Geometry: see drawing. Coordinates: mm, zero at the bounding-box minimum. A direction names the side the tool comes from. Coordinates: 2 decimals unless noted, no trailing zeros. Loops run counter-clockwise (first coordinate to the right, second up) from the corner with the lowest first, then second, coordinate; pieces in that order, holes last. Notation, with made-up numbers: (-9, -34.5) -> (46, -34.5) arc R14 ccw to (46, -20.5) -> close; hole circle Ø4 at (-13.75, 59). An arc over 180 degrees is marked (long way). One line per item, written item: value. Start each with the question number.
Item 1: Section query A-A on z = 3.35. Return loops of the section in (x, y).
Item 2: Ray query, probe 1 along Y at (x, z) = (4.75, 1.75); probe 2 along Y at (x, z) = (4.25, 3.5); probe 3 along Z at (x, y) = (5, 2). Return the intervals inside material, ascending. Write a range as from..to.
Item 3: Set-up query: the marked faces 1 and 2. Return all of +Z, -Z, +X, -X, +Y, -Y with unobstructed straight access to the full face (end or side cutting, diameter ignored); none if empty.
Item 4: Contact query for flat-ended pins moving along their axis: pin 1 Ø0.5 at (y, z) = (14, 4) entering from +X; pin 2 Ø1 at (x, y) = (2.5, 4.5) entering from -Z; pin 3 Ø0.6 at (y, z) = (14.5, 3.5) entering from +X. Output: stop coordinate, or through.
Item 5: Section query B-B on y = 8.75. Return loops of the section in (x, z).
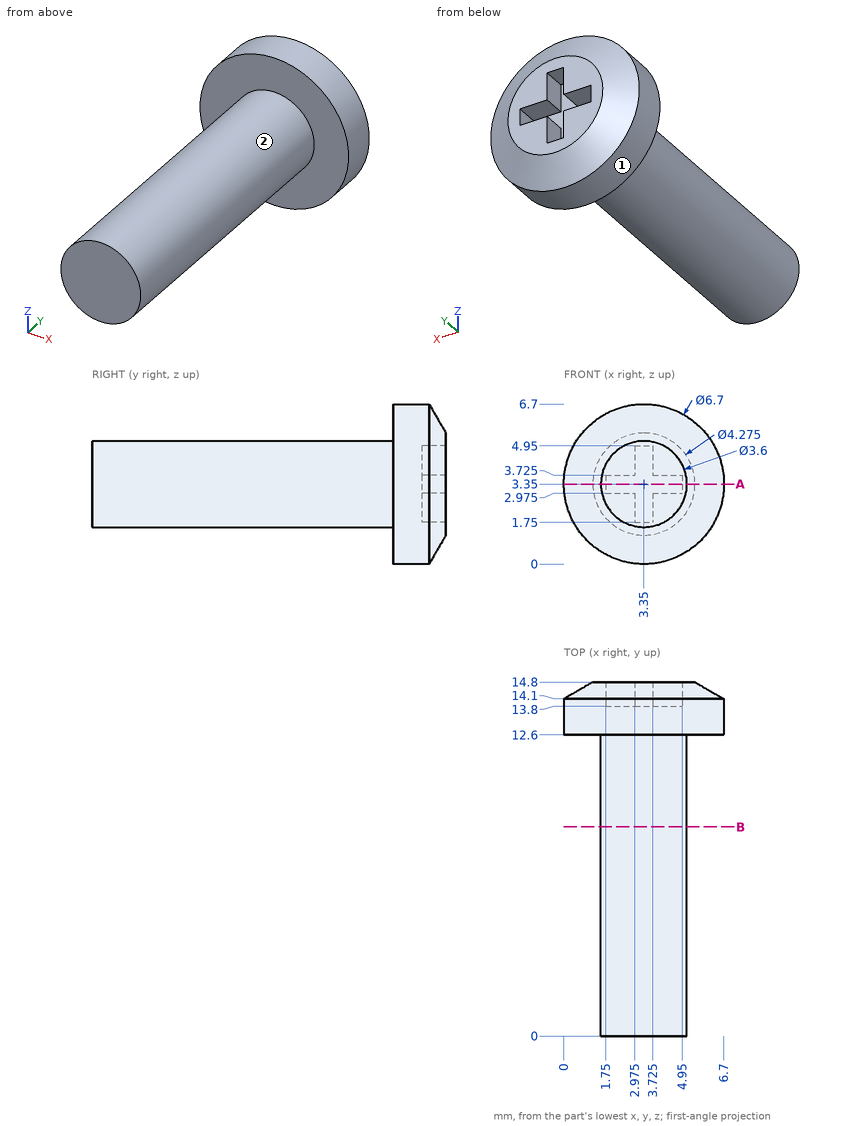
Reply:
1. outline: (0, 12.6) -> (1.55, 12.6) -> (1.55, 0) -> (5.15, 0) -> (5.15, 12.6) -> (6.7, 12.6) -> (6.7, 14.1) -> (5.49, 14.8) -> (4.95, 14.8) -> (4.95, 13.8) -> (1.75, 13.8) -> (1.75, 14.8) -> (1.21, 14.8) -> (0, 14.1) -> close
2. probe 1: y = 12.6..14.8
2. probe 2: y = 0..13.8
2. probe 3: z = 2.63..4.07
3. face 1: +Y, -Y
3. face 2: -Y
4. pin 1: stops at x = 6.68
4. pin 2: stops at z = 1.58
4. pin 3: stops at x = 6.52
5. outline: circle Ø3.6 at (3.35, 3.35)
